Geometry: final body of the model. Coordinates: model frame, mm. Face numbers are marked on the shaded views. Coordinates: 2 decimals unless noted, no trailing zeros. Loops run counter-clockwise (first coordinate to the right, second up) from the corner with the lowest first, then second, coordinate; pieces in that order, holes last. Notation, with made-up numbers: (67, 43) - (103, 43) arc R13 cw to (103, 54) - close; hole circle Ø4 at (74, -31). An arc over 180 degrees is marked (long way). Return JSON: item names as keys, results as strings.
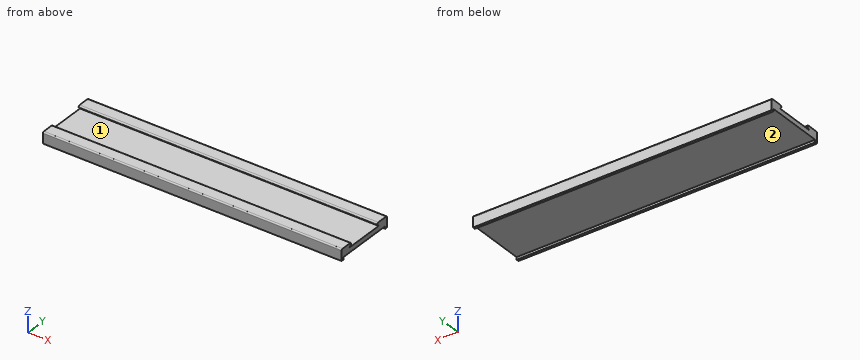
from build123d import *

# Parameters (mm, degrees)
SKETCH1_W           = 120
SKETCH1_H           = 25
BOSS_EXTRUDE1_DEPTH = 3.5
SKETCH1_3_W         = 120
SKETCH1_3_H         = 1
BOSS_EXTRUDE2_DEPTH = 1
CUT_EXTRUDE1_DEPTH  = 121
FILLET1_R           = 0.5
FILLET2_R           = 0.5


with BuildPart() as part:
    # Sketch1 → Boss-Extrude1 (new body)
    with BuildSketch(Plane.XY):
        with Locations((60, 12.5)):
            Rectangle(SKETCH1_W, SKETCH1_H)
    extrude(amount=BOSS_EXTRUDE1_DEPTH)

    # Sketch1<3> → Boss-Extrude2 (add)
    with BuildSketch(Plane.XY):
        with Locations((60, 24.5)):
            Rectangle(SKETCH1_3_W, SKETCH1_3_H)
        with Locations((60, 0.5)):
            Rectangle(SKETCH1_3_W, SKETCH1_3_H)
    extrude(amount=-BOSS_EXTRUDE2_DEPTH)

    # Sketch3 → Cut-Extrude1 (cut, through all)
    with BuildSketch(Plane(origin=(120, 0, 0), x_dir=(0, 0, -1), z_dir=(1, 0, 0))):
        Polygon((-2, 20.384047046), (-3.5, 19), (-3.5, 6), (-2, 4.374332717), align=None)
    extrude(amount=-CUT_EXTRUDE1_DEPTH, mode=Mode.SUBTRACT)

    # Fillet1
    fillet1_edges = [part.edges().sort_by_distance(p)[0] for p in [
        (60, 19, 3.5),
        (60, 6, 3.5),
    ]]
    fillet(fillet1_edges, radius=FILLET1_R)

    # Fillet2
    fillet2_edges = [part.edges().sort_by_distance(p)[0] for p in [
        (60, 0, 3.5),
        (60, 25, 3.5),
    ]]
    fillet(fillet2_edges, radius=FILLET2_R)


solid = part.part
Item 1: Mould query, pull axis Y, two halves, no side actions, for the marked faces 1 and 2. Classes: +Y half, -Y half, draft (parallel to the pull), parting line (faces both ways), or undercut.
Worked out:
{"face 1": "undercut", "face 2": "undercut"}
Item 2: Section query A-A, the plane x = 77. Return loops of the section in (y, z).
Worked out:
{"outline": "(0, -1) - (1, -1) - (1, 0) - (24, 0) - (24, -1) - (25, -1) - (25, 3) arc R0.5 ccw to (24.5, 3.5) - (20.14, 3.5) arc R0.5 ccw to (19.77, 2.66) - (20.38, 2) - (4.37, 2) - (5.06, 2.63) arc R0.5 ccw to (4.72, 3.5) - (0.5, 3.5) arc R0.5 ccw to (0, 3) - close"}
Item 3: Section query B-B, the plane y = 14. Return loops of the section in (x, z), and give its area (3 significant figures).
Worked out:
{"outline": "(0, 0) - (120, 0) - (120, 2) - (0, 2) - close", "area": "240 mm^2"}
Item 4: Ray query, probe 1 along Y at (x, z) = (62, 3.05); probe 2 along Y at (x, z) = (46.5, 3.1); probe 3 along Z at (x, y) = (95.5, 22.75). Return the intervals inside material, ascending. Write a range as from..to.
Worked out:
{"probe 1": "0..5.22, 19.64..25", "probe 2": "0.01..5.21, 19.65..24.99", "probe 3": "0..3.5"}
Item 5: First-contact query: pin 1 Ø5 at (x, y) = (95, 8) entering from -Z; pin 2 Ø2 at (y, z) = (9.5, 0.5) entering from -X. Flat tips, straight axial feed; report the tip coordinate or a pass-through.
Worked out:
{"pin 1": "z = 0", "pin 2": "x = 0"}
